CAD build for the part. Positions are in the model's coordinates, mm. A direction names the side the tool comes from. Round coordinates to 2 decimals unless told otherwise and drop trailing zeros. Loops run counter-clockwise (first coordinate to the right, second up) from the corner with the lowest first, then second, coordinate; pieces in that order, holes last.
Autodesk Fusion 360 part; units mm, degrees
sketch "Sketch1" plane through (0, 0, 0) normal (0, 0, 1) x (1, 0, 0)
  line L0 (0, 0) -> (117.82, 0)
  line L1 (117.82, 0) -> (117.82, 72.6)
  line L2 (117.82, 72.6) -> (0, 72.6)
  line L3 (0, 72.6) -> (0, 0)
  circle A0 centre (10.6, 67.88) radius 1.4
  circle A1 centre (10.6, 4.78) radius 1.4
  circle A2 centre (105.7, 67.88) radius 1.4
  line L4 (10.6, 67.88) -> (10.6, 69.28) construction
  line L5 (105.7, 67.88) -> (105.7, 69.28) construction
  line L6 (10.6, 67.88) -> (9.2, 67.88) construction
  line L7 (105.7, 67.88) -> (107.1, 67.88) construction
  line L8 (10.6, 4.78) -> (10.6, 3.38) construction
  line L9 (10.6, 4.78) -> (9.2, 4.78) construction
  line L10 (10.6, 67.88) -> (105.7, 67.88) construction
  line L11 (10.6, 67.88) -> (10.6, 4.78) construction
  line L12 (0, 36.3) -> (117.82, 36.3) construction
  circle A3 centre (3, 36.3) radius 1.5
  circle A4 centre (115.12, 36.3) radius 1.5
  dimension "d1" = 117.82
  dimension "d2" = 72.6
  dimension "d3" = 2.8
  dimension "d4" = 2.8
  dimension "d6" = 2.8
  dimension "d18" = 95.1
  dimension "d19" = 63.1
  dimension "d20" = 4.72
  dimension "d21" = 10.6
  dimension "d22" = 3
  dimension "d23" = 3
  dimension "d24" = 2.7
  dimension "d25" = 3
sketch "Sketch2" plane through (0, 0, 0) normal (0, 0, -1) x (1, 0, 0)
  circle A0 centre (10.6, -67.88) radius 1.4
  circle A1 centre (105.7, -67.88) radius 1.4
  circle A2 centre (10.6, -4.78) radius 1.4
  line L0 (0, 0) -> (0, -72.6)
  line L1 (0, -72.6) -> (117.82, -72.6)
  line L2 (117.82, -72.6) -> (117.82, 0)
  line L3 (117.82, 0) -> (0, 0)
  line L4 (117.82, -72.6) -> (0, 0) construction
  line L5 (0, -72.6) -> (117.82, 0) construction
  line L6 (88.1333, -48) -> (51.3806, -48)
  line L7 (51.3806, -48) -> (51.3806, -6)
  line L8 (51.3806, -6) -> (88.1333, -6)
  line L9 (88.1333, -6) -> (88.1333, -48)
  circle A3 centre (3, -36.3) radius 1.5
  circle A4 centre (115.12, -36.3) radius 1.5
sketch "Sketch3" plane through (0, 0, 1.5) normal (0, 0, 1) x (-1, 0, 0)
  circle A0 centre (-10.6, -67.88) radius 1.4
  circle A1 centre (-105.7, -67.88) radius 1.4
  circle A2 centre (-10.6, -4.78) radius 1.4
  circle A3 centre (-3, -36.3) radius 1.5
  circle A4 centre (-115.12, -36.3) radius 1.5
  line L0 (0, -72.6) -> (0, 0)
  line L1 (0, 0) -> (-117.82, 0)
  line L2 (-117.82, 0) -> (-117.82, -72.6)
  line L3 (-117.82, -72.6) -> (0, -72.6)
  line L4 (-6.41, -73) -> (-111.41, -73)
  line L5 (-111.41, -73) -> (-111.41, 0)
  line L6 (-111.41, 0) -> (-6.41, 0)
  line L7 (-6.41, 0) -> (-6.41, -73)
  line L8 (-6.41, -41.1844) -> (-0.01, -41.1844)
  line L9 (-0.01, -41.1844) -> (-0.01, -31.8156)
  line L10 (-0.01, -31.8156) -> (-6.41, -31.8156)
  line L11 (-111.41, -40.5951) -> (-117.27, -40.5951)
  line L12 (-117.27, -40.5951) -> (-117.27, -32.0049)
  line L13 (-117.27, -32.0049) -> (-111.41, -32.0049)
  line L14 (-117.27, -36.3) -> (-111.41, -36.3) construction
  line L15 (-0.01, -36.5) -> (-6.41, -36.5) construction
  line L16 (-58.91, 0) -> (-58.91, -72.6) construction
  point P0 (-115.12, -36.3)
  point P1 (-3, -36.5)
  dimension "d26" = 105
  dimension "d27" = 73
  dimension "d30" = 6.4
  dimension "d31" = 117.26
extrude "Extrude3" add sketch "Sketch3" along normal blind 22 contours A0 | A1 | A2 | L1 L3 L5 L6 L7
extrude "Extrude4" add sketch "Sketch3" along normal blind 2 contours L7 L8 L9 L10 | L5 L11 L12 L13
chamfer "Chamfer1" distance 5 angle 45 3 edges at (6.41, 36.3, 23.5) (58.91, 72.6, 23.5) (111.41, 36.3, 23.5)
shell "Shell1" thickness 2 removed faces 1 at (43.0767, 0, 8.8333)
extrude "Extrude5" cut sketch "Sketch1" along normal blind 3.5 contours A0 | A1 | A2
equation "d4 = d3"
equation "d6 = d3"
equation "d18 = 92.3 mm + d3"
equation "d19 = 60.3 mm + d3"
Item 1: Cut at C-C, the plane y = 4.78. Give the cut face in (x, z), plus the area to 3 significant figures.
Answers follow:
outline: (6.41, 1.5) - (9.2, 1.5) - (9.2, 3.5) - (12, 3.5) - (12, 1.5) - (111.41, 1.5) - (111.41, 18.5) - (106.41, 23.5) - (11.41, 23.5) - (6.41, 18.5) - close
area: 2,280 mm2
Item 2: Cut at A-A, the plane y = 36.3. Give the cut face in (x, z), plus the area to 3 significant figures.
Answers follow:
outline: (0.01, 1.5) - (1.5, 1.5) - (1.5, 3.5) - (0.01, 3.5) - close; (4.5, 1.5) - (113.62, 1.5) - (113.62, 3.5) - (111.41, 3.5) - (111.41, 18.5) - (106.41, 23.5) - (11.41, 23.5) - (6.41, 18.5) - (6.41, 3.5) - (4.5, 3.5) - close; (116.62, 1.5) - (117.27, 1.5) - (117.27, 3.5) - (116.62, 3.5) - close
area: 2,300 mm2
Item 3: Cut at B-B, the plane x = 3. Give the cut face in (y, z).
Answers follow:
outline: (31.82, 1.5) - (34.8, 1.5) - (34.8, 3.5) - (31.82, 3.5) - close; (37.8, 1.5) - (41.18, 1.5) - (41.18, 3.5) - (37.8, 3.5) - close
Item 4: 3-axis set-ups, long thin cutter, end or side, ignore diameter. For faces 4 (the flat face through (60, 33, 23.5)), 5 (the flat face through (114, 35, 3.5)), 6 (the flat face through (11, 68, 3.5)), 7 (the flat face through (5, 36, 3.5)): which of +Z, -Z, +X, -X, +Y, -Y reach the whole face in a straight line?
Answers follow:
face 4: +Z, +X, -X, +Y, -Y
face 5: +Z, +X, +Y, -Y
face 6: -Z
face 7: +Z, -X, +Y, -Y
Item 5: Two-plate mould, pull along Y, no slides. Class faces 1 (the cylindrical face through (104.3, 67.82, 2.49)), 2 (the flat face through (6.41, 36, 10)), 3 (the flat face through (58.2, 70.1, 21)): released by +Y, released by -Y, zero draft, split by the parting line, or undercut.
Answers follow:
face 1: undercut
face 2: zero draft
face 3: released by +Y
Item 6: Flat gauge pins, fed straight in: P1, Ø2.5, axis at x = 105.7, y = 67.88, coming from the +Z side; P2, Ø2, axis at x = 3.5, z = 2.5, coming from the -Y side; P3, Ø2, axis at x = 115, z = 2.5, coming from the +Y side; P4, Ø1.4, axis at x = 11, y = 68, coming from the -Z side. Where does each tip first touch, or does it go through?
Answers follow:
P1: stops at z = 23.5
P2: stops at y = 31.82
P3: stops at y = 40.6
P4: stops at z = 3.5
Item 7: Probe line 1 (Y direction, x = 10.6, z = 2.1); line 2 (X direction, y = 67.88, z = 2.55); line 3 (X direction, y = 36.3, z = 2.8). List the from-to ranges inside material, lowest first.
Answers follow:
line 1: y = 0 to 3.38, 6.18 to 66.48, 69.28 to 72.6
line 2: x = 6.41 to 9.2, 12 to 104.3, 107.1 to 111.41
line 3: x = 0.01 to 1.5, 4.5 to 113.62, 116.62 to 117.27
Item 8: Cut at D-D, the plane x = 115.12. Give the cut face in (y, z), plus the area to 3 significant figures.
Answers follow:
outline: (32, 1.5) - (34.8, 1.5) - (34.8, 3.5) - (32, 3.5) - close; (37.8, 1.5) - (40.6, 1.5) - (40.6, 3.5) - (37.8, 3.5) - close
area: 11.2 mm2
